The model under review builds one solid part; all positions refer to its coordinate system, in mm. Coordinates: 2 decimals unless noted, no trailing zeros. Order: outer loops, then holes, each group sorted by start corner. A loop starts at its lowest first (then second) coordinate and runs counter-clockwise, first axis right, second up. Notation, with made-up numbers: M 88.5,-25 L 111.5,-25 A21 ccw 111.5,-20 Z; hole C 6,82 d6. An arc over 180 degrees is marked long. One line per item, written item: value.
```python
from build123d import *

# Parameters (mm, degrees)
F0_R     = 12.7
F1_DEPTH = 152.4
F2_R     = 1.8796
F3_DEPTH = 25.4
F4_R     = 1.8796
F5_DEPTH = 25.4


with BuildPart() as f1:
    # F0 (on Top) → F1 (new body)
    with BuildSketch(Plane.XY):
        Circle(F0_R)
    extrude(amount=F1_DEPTH)

    # F2 (on Front) → F3 (cut, symmetric)
    with BuildSketch(Plane.XZ):
        with Locations((0, 12.7)):
            Circle(F2_R)
    extrude(amount=F3_DEPTH, both=True, mode=Mode.SUBTRACT)

    # F4 (on Front) → F5 (cut, symmetric)
    with BuildSketch(Plane.XZ):
        with Locations((0, 139.7)):
            Circle(F4_R)
    extrude(amount=F5_DEPTH, both=True, mode=Mode.SUBTRACT)


solid = f1.part
```
(1) We need section B-B, the plane y = 10. State the section outline as (x, z) points, plus the area to 3 significant figures.
Geometry results:
outline: M -7.83,0 L 7.83,0 L 7.83,152.4 L -7.83,152.4 Z; hole C 0,12.7 d3.76; hole C 0,139.7 d3.76
area: 2,360 mm2
(2) Insertion check: pin 1 Ø8 at (x, z) = (-7, 73) entering from +Y; pin 2 Ø3 at (x, z) = (0, 12.7) entering from +Y; pin 3 Ø2 at (x, z) = (-5.5, 57) entering from +Y; pin 4 Ø2 at (x, z) = (9.5, 118) entering from +Y. Each pin has a flat end and moves straight along its axis. Give the tip position at first contact, or say it passes through.
Geometry results:
pin 1: stops at y = 12.34
pin 2: passes through
pin 3: stops at y = 11.88
pin 4: stops at y = 9.44
(3) We need section C-C, the plane z = 49.5. State the section outline as (x, y) points.
Geometry results:
outline: C 0,0 d25.4
(4) For L1, parallel to Z at x = 0, y = 4.75; L2, parallel to X at y = 3.25, z = 139.7; L3, parallel to X at y = 7.25, z = 139.7, list the stretches that pass through material, from the lowest coordinate up.
Geometry results:
L1: z = 0 to 10.82, 14.58 to 137.82, 141.58 to 152.4
L2: x = -12.28 to -1.88, 1.88 to 12.28
L3: x = -10.43 to -1.88, 1.88 to 10.43
(5) Mouldability with a two-part tool opening along X and no side actions: class faces 1 (the cylindrical face through (-2.75, -12.4, 75.13)), 2 (the flat face through (0, 0, 0)), 3 (the cylindrical face through (-1.385, -0.178, 13.97)) as +X half, -X half, draft (parallel to the pull), parting line (faces both ways), or undercut.
Geometry results:
face 1: parting line
face 2: draft
face 3: undercut
(6) We need section A-A, the plane x = 0. State the section outline as (y, z) points.
Geometry results:
outline: M -12.7,0 L 12.7,0 L 12.7,10.82 L -12.7,10.82 Z; M -12.7,14.58 L 12.7,14.58 L 12.7,137.82 L -12.7,137.82 Z; M -12.7,141.58 L 12.7,141.58 L 12.7,152.4 L -12.7,152.4 Z
(7) We need section D-D, the plane z = 139.7. State the section outline as (x, y) points.
Geometry results:
outline: M -1.88,-12.56 L -1.88,12.56 A12.7 ccw Z; M 1.88,-12.56 A12.7 ccw 1.88,12.56 Z
